Design review of the part built by this model. Coordinates are the model's own, in mm. Coordinates: 2 decimals unless noted, no trailing zeros. Order: outer loops, then holes, each group sorted by start corner. A loop starts at its lowest first (then second) coordinate and runs counter-clockwise, first axis right, second up. Notation, with made-up numbers: (36, 57) -> (91, 57) arc R13 ccw to (91, 62) -> close; hole circle Ø6 at (-3.5, 72). An arc over 180 degrees is marked (long way). Use a Markdown table: item, result. Add a question column.
Q1. Add section C-C (z = 1). Count the separate pieces of the cut face and the enclosed holes in it, then the cut area to 3 significant figures.
Q2. Add section A-A (y = 8). State the section outline as (x, z) points, then the cut area to 3 significant figures.
Q3. Add section B-B (x = 24.5). State the section outline as (y, z) points, then the cut area to 3 significant figures.
Q4. Insertion check: pin 1 (0.9 mm diameter, centred on x = 74, z = 1.5, fed in from +Y); pin 2 (1.5 mm diameter, centred on x = 35.5, z = 2.5, fed in from +Y); pin 3 (1.5 mm diameter, centred on x = 45.74, y = 18.03, fed in from +Z); pin 4 (1.5 mm diameter, centred on y = 14, z = 1.5, fed in from -X). Each pin has a flat end and moves straight along its axis. Give the tip position at first contact, or say it passes through.
Q5. Add section D-D (y = 36). State the section outline as (x, z) points, then the cut area to 3 significant figures.
Q6. Wall thickness on probe 1 along X at (y, z) = (72.5, 2.05); probe 2 along X at (y, z) = (11.5, 1.25); probe 3 along X at (y, z) = (52.5, 1.1): over which ranges is each line inside the solid? List them lowest first.
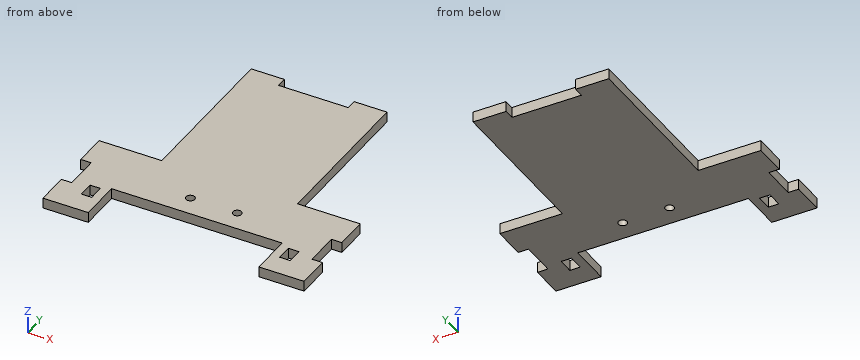
from build123d import *

# Parameters (mm, degrees)
SALIENTE_EXTRUIR1_DEPTH = 3
CROQUIS4_W              = 49
CROQUIS4_H              = 12
CORTAR_EXTRUIR2_DEPTH   = 10
CROQUIS5_R              = 1.25
CORTAR_EXTRUIR3_DEPTH   = 10
CROQUIS6_W              = 3
CROQUIS6_H              = 4.5
CORTAR_EXTRUIR4_DEPTH   = 10


with BuildPart() as part:
    # Croquis1 → Saliente-Extruir1 (new body)
    with BuildSketch(Plane.XY):
        Polygon((0, 28.9), (18, 28.9), (18, 75), (27.5, 75), (27.5, 72), (47.5, 72), (47.5, 75), (57, 75), (57, 28.9), (75, 28.9), (75, 19.45), (72, 19.45), (72, 9.45), (75, 9.45), (75, 0), (0, 0), (0, 9.45), (3, 9.45), (3, 19.45), (0, 19.45), align=None)
    extrude(amount=SALIENTE_EXTRUIR1_DEPTH)

    # Croquis4 → Cortar-Extruir2 (cut)
    with BuildSketch(Plane.XY.offset(3)):
        with Locations((37.5, 6)):
            Rectangle(CROQUIS4_W, CROQUIS4_H)
    extrude(amount=-CORTAR_EXTRUIR2_DEPTH, mode=Mode.SUBTRACT)

    # Croquis5 → Cortar-Extruir3 (cut)
    with BuildSketch(Plane(origin=(0, 0, 0), x_dir=(-1, 0, 0), z_dir=(0, 0, -1))):
        with Locations((-32.279739901, 18.033331943)):
            Circle(CROQUIS5_R)
        with Locations((-45.741739901, 18.033331943)):
            Circle(CROQUIS5_R)
    extrude(amount=-CORTAR_EXTRUIR3_DEPTH, mode=Mode.SUBTRACT)

    # Croquis6 → Cortar-Extruir4 (cut)
    with BuildSketch(Plane(origin=(0, 0, 0), x_dir=(-1, 0, 0), z_dir=(0, 0, -1))):
        with Locations((-9, 8.5)):
            Rectangle(CROQUIS6_W, CROQUIS6_H)
        with Locations((-66, 8.5)):
            Rectangle(CROQUIS6_W, CROQUIS6_H)
    extrude(amount=-CORTAR_EXTRUIR4_DEPTH, mode=Mode.SUBTRACT)


solid = part.part
Established:
| question | item | result |
|---|---|---|
| 1 | separate pieces | 1 |
| 1 | enclosed holes | 4 |
| 1 | area | 3,220 mm^2 |
| 2 | outline | (0, 0) -> (7.5, 0) -> (7.5, 3) -> (0, 3) -> close; (10.5, 0) -> (13, 0) -> (13, 3) -> (10.5, 3) -> close; (62, 0) -> (64.5, 0) -> (64.5, 3) -> (62, 3) -> close; (67.5, 0) -> (75, 0) -> (75, 3) -> (67.5, 3) -> close |
| 2 | area | 60.0 mm^2 |
| 3 | outline | (12, 0) -> (75, 0) -> (75, 3) -> (12, 3) -> close |
| 3 | area | 189 mm^2 |
| 4 | pin 1 | y = 28.9 |
| 4 | pin 2 | y = 72 |
| 4 | pin 3 | through |
| 4 | pin 4 | x = 3 |
| 5 | outline | (18, 0) -> (57, 0) -> (57, 3) -> (18, 3) -> close |
| 5 | area | 117 mm^2 |
| 6 | probe 1 | 18 to 27.5, 47.5 to 57 |
| 6 | probe 2 | 3 to 13, 62 to 72 |
| 6 | probe 3 | 18 to 57 |
